from build123d import *

# Parameters (mm, degrees)
SKETCH1_W               = 54
SKETCH1_H               = 35
BOSS_EXTRUDE1_DEPTH     = 10
SKETCH2_W               = 22
SKETCH2_H               = 10
CUT_EXTRUDE1_DEPTH      = 29
SKETCH3_W               = 22
SKETCH3_H               = 10
CUT_EXTRUDE2_DEPTH      = 15
SKETCH5_R               = 1.45
CUT_EXTRUDE4_DEPTH      = 66.122960621
FILLET1_R               = 3
FILLET2_R               = 3
SKETCH8_W               = 10
SKETCH8_H               = 10
BOSS_EXTRUDE2_DEPTH     = 3
CUT_EXTRUDE5_DEPTH      = 4
CUT_EXTRUDE5_DEPTH_BACK = 15
SKETCH6_R               = 1.45
FILLET3_R               = 4


with BuildPart() as part:
    # Sketch1 → Boss-Extrude1 (new body)
    with BuildSketch(Plane(origin=(0, 0, 0), x_dir=(1, 0, 0), z_dir=(0, 1, 0))):
        with Locations((27, -17.5)):
            Rectangle(SKETCH1_W, SKETCH1_H)
    extrude(amount=BOSS_EXTRUDE1_DEPTH)

    # Sketch2 → Cut-Extrude1 (cut)
    with BuildSketch(Plane(origin=(54, 0, 0), x_dir=(0, 0, -1), z_dir=(1, 0, 0))):
        with Locations((-17.5, 5)):
            Rectangle(SKETCH2_W, SKETCH2_H)
    extrude(amount=-CUT_EXTRUDE1_DEPTH, mode=Mode.SUBTRACT)

    # Sketch3 → Cut-Extrude2 (cut)
    with BuildSketch(Plane.ZY):
        with Locations((17.5, 5)):
            Rectangle(SKETCH3_W, SKETCH3_H)
    extrude(amount=-CUT_EXTRUDE2_DEPTH, mode=Mode.SUBTRACT)

    # Sketch5 → Cut-Extrude4 (cut, through all)
    with BuildSketch(Plane.XY.offset(35)):
        with Locations((5, 5)):
            Circle(SKETCH5_R)
        with Locations((49, 5)):
            Circle(SKETCH5_R)
    extrude(amount=-CUT_EXTRUDE4_DEPTH, mode=Mode.SUBTRACT)

    # Fillet1
    fillet1_edges = [part.edges().sort_by_distance(p)[0] for p in [
        (54, 10, 31.75),
        (54, 0, 3.25),
        (54, 10, 3.25),
        (0, 0, 31.75),
        (0, 10, 31.75),
        (0, 10, 3.25),
        (54, 0, 31.75),
        (0, 0, 3.25),
    ]]
    fillet(fillet1_edges, radius=FILLET1_R)

    # Fillet2
    fillet2_edges = [part.edges().sort_by_distance(p)[0] for p in [
        (25, 5, 28.5),
        (25, 5, 6.5),
        (15, 5, 6.5),
        (15, 5, 28.5),
    ]]
    fillet(fillet2_edges, radius=FILLET2_R)

    # Sketch8 → Boss-Extrude2 (add)
    with BuildSketch(Plane.XY.offset(35)):
        with Locations((20, 5)):
            Rectangle(SKETCH8_W, SKETCH8_H)
    extrude(amount=BOSS_EXTRUDE2_DEPTH)

    # Sketch6 → Cut-Extrude5 (cut, two sides: drawn at the far end of the back side and taken through both)
    with BuildSketch(Plane.XY.offset(35).offset(-CUT_EXTRUDE5_DEPTH_BACK)):
        with Locations((19.5, 5)):
            Circle(SKETCH6_R)
    extrude(amount=CUT_EXTRUDE5_DEPTH + CUT_EXTRUDE5_DEPTH_BACK, mode=Mode.SUBTRACT)

    # Fillet3
    # the kernel refuses this fillet: 4 mm, written as the material it adds along each edge
    with BuildSketch(Plane(origin=(25, 10, 35), x_dir=(0, 0, 1), z_dir=(0, -1, 0))) as fillet3_piece_1:
        with BuildLine():
            CenterArc((4, -3.872983346), FILLET3_R, 104.477512186, 75.522487814)
            Line((0, -3.872983346), (-0.08, -3.872983346))
            Line((-0.08, -3.872983346), (-0.08, 0))
            Line((-0.08, 0), (0, 0.08))
            ThreePointArc((0, 0.08), (1.5, 0.08), (2.98, 0.077459667))
            Line((2.98, 0.077459667), (3, 0))
        make_face()
    extrude(amount=10)
    with BuildSketch(Plane(origin=(15, 0, 35), x_dir=(-1, 0, 0), z_dir=(0, 1, 0))) as fillet3_piece_2:
        with BuildLine():
            CenterArc((3.872983346, 4), FILLET3_R, 194.477512186, 75.522487814)
            Line((0, 3), (-0.077459667, 2.98))
            ThreePointArc((-0.077459667, 2.98), (-0.08, 1.5), (-0.08, 0))
            Line((-0.08, 0), (0, -0.08))
            Line((0, -0.08), (3.872983346, -0.08))
            Line((3.872983346, -0.08), (3.872983346, 0))
        make_face()
    extrude(amount=10)


solid = part.part
Verification items for the finished model (mm, model axes). A direction names the side the tool comes from. Give positions to 0.01 mm unless a question says otherwise; leave off trailing zeros. Write each loop counter-clockwise with the first axis right and the second up, starting at its lowest first coordinate (ties: lowest second). Pieces come first, ordered by that corner, then holes.
(1) Cross-section at D-D (y = 7.75). Enter the section's corners in (x, z), plus the area to 3 significant figures.
(2) Gauge pin test, flat ends, axial feed: pin 1 (5 mm diameter, centred on x = 37, y = 5.5, fed in from -Z); pin 2 (4.5 mm diameter, centred on x = 5, y = 5, fed in from +Z); pin 3 (5 mm diameter, centred on y = 5, z = 14.5, fed in from -X); pin 4 (2 mm diameter, centred on y = 4.5, z = 21, fed in from +X). Record the tip position at first contact, or that the pin passes through.
(3) Cross-section at A-A (x = 30.5). Enter the section's corners in (y, z), plus the area to 3 significant figures.
(4) Mould release check, pull along Y, two halves, no side actions. Record for faces 5 (the face through (53.1, 9.14, 3.2)), 6 (the face through (20.88, 5.44, 28.87)), 7 (the face through (0.9, 0.86, 3.2)), 8 (the face through (7, 5, 35)): +Y half, -Y half, draft (parallel to the pull), parting line (faces both ways), or undercut.
(5) Cross-section at B-B (z = 32). Enter the section's corners in (x, y).
(6) Material ranges on line 1 (Z direction, x = 44, y = 9); line 2 (Y direction, x = 5, z = 32); line 3 (X direction, y = 8.5, z = 13), recorded low to high.
(7) Cross-section at C-C (x = 49). Enter the section's corners in (y, z).
(8) Access from +Z, -Z, +X, -X, +Y, -Y to the whole of each face (thin tool, end or side, straight path). Record for faces 1 (the face through (19, 5, 20)), 2 (the face through (15, 5, 17)), 3 (the face through (53.1, 0.86, 3.2)), 4 (the face through (25.86, 5.07, 7.4)).
Worked out:
1. outline: (0.1, 0) - (53.9, 0) - (53.9, 6.5) - (28, 6.5) arc R3 cw to (25, 9.5) - (25, 25.5) arc R3 cw to (28, 28.5) - (53.9, 28.5) - (53.9, 35) - (28.87, 35) arc R4 cw to (25, 38) - (15, 38) arc R4 cw to (11.13, 35) - (0.1, 35) - (0.1, 28.5) - (12, 28.5) arc R3 cw to (15, 25.5) - (15, 9.5) arc R3 cw to (12, 6.5) - (0.1, 6.5) - close
1. area: 963 mm2
2. pin 1: stops at z = 0
2. pin 2: stops at z = 35
2. pin 3: stops at x = 15
2. pin 4: stops at x = 25
3. outline: (0, 0) - (10, 0) - (10, 6.5) - (0, 6.5) - close; (0, 28.5) - (10, 28.5) - (10, 35) - (0, 35) - close
3. area: 130 mm2
4. face 5: +Y half
4. face 6: undercut
4. face 7: -Y half
4. face 8: draft
5. outline: (0, 3) arc R3 ccw to (3, 0) - (51, 0) arc R3 ccw to (54, 3) - (54, 7) arc R3 ccw to (51, 10) - (3, 10) arc R3 ccw to (0, 7) - close; hole circle Ø2.9 at (5, 5); hole circle Ø2.9 at (19.5, 5); hole circle Ø2.9 at (49, 5)
6. line 1: z = 0 to 6.5, 28.5 to 35
6. line 2: y = 0 to 3.55, 6.45 to 10
6. line 3: x = 15 to 25
7. outline: (0, 0) - (3.55, 0) - (3.55, 6.5) - (0, 6.5) - close; (0, 28.5) - (3.55, 28.5) - (3.55, 35) - (0, 35) - close; (6.45, 0) - (10, 0) - (10, 6.5) - (6.45, 6.5) - close; (6.45, 28.5) - (10, 28.5) - (10, 35) - (6.45, 35) - close
8. face 1: +Z
8. face 2: -X, +Y, -Y
8. face 3: +Z, -Z, +X, -Y
8. face 4: +X, +Y, -Y
